```python
from build123d import *

# Parameters (mm, degrees)
CUT_EXTRUDE1_DEPTH = 3.5
CHAMFER1_SIZE      = 0.288675135
CHAMFER1_SIZE2     = 0.5


with BuildPart() as part:
    # Sketch1 → Revolve1 (revolve)
    with BuildSketch(Plane.XY, mode=Mode.PRIVATE) as revolve1_sk:
        Polygon((-20, 2), (-19, 3), (0, 3), (0, 0), (-20, 0), align=None)
    revolve(revolve1_sk.sketch.rotate(Axis((0, 0, 0), (-1, 0, 0)), 90), axis=Axis((0, 0, 0), (-1, 0, 0)))

    # Sketch2 → Cut-Extrude1 (cut)
    with BuildSketch(Plane(origin=(0, 0, 0), x_dir=(0, 0, -1), z_dir=(1, 0, 0))):
        Polygon((1.732050808, 0), (0.866025404, 1.5), (-0.866025404, 1.5), (-1.732050808, 0), (-0.866025404, -1.5), (0.866025404, -1.5), align=None)
    extrude(amount=-CUT_EXTRUDE1_DEPTH, mode=Mode.SUBTRACT)

    # Chamfer1
    chamfer1_edges = [part.edges().sort_by_distance(p)[0] for p in [
        (0, 0, 3),
    ]]
    chamfer1_side = [part.faces().sort_by_distance(p)[0] for p in [
        (-9.5, 0, 3),
    ]]
    chamfer(chamfer1_edges, length=CHAMFER1_SIZE, length2=CHAMFER1_SIZE2, reference=chamfer1_side[0])


solid = part.part
```
Could you check a few things on this model? Use its own coordinates, in mm. A direction names the side the tool comes from. Coordinates: 2 decimals unless noted, no trailing zeros. Write each loop counter-clockwise with the first axis right and the second up, starting at its lowest first coordinate (ties: lowest second). Pieces come first, ordered by that corner, then holes. Notation, with made-up numbers: (11.25, -6) -> (22.25, -6) arc R16 ccw to (22.25, 24) -> close; hole circle Ø1 at (71, 49.5). An arc over 180 degrees is marked (long way). Write item = value, one per line. Start each with the question number.
(1) We'd pull the mould along Z, two halves only. Please class faces 1 (the face through (0, 2, 0)), 2 (the face through (-9.51, -0.9, -2.86)), 3 (the face through (-1.726, 0.76, 1.293)): released by +Z, released by -Z, zero draft, split by the parting line, or undercut.
(2) Which directions (+Z, -Z, +X, -X, +Y, -Y) give clear straight access to the entire face, cutting with the end or side of a thin tool? Please do faces 4 (the face through (-20, 0, 0)), 5 (the face through (-2, -1.5, 0)).
(3) I want a section at C-C (x = -8.75). Please give me the cut outline in (y, z).
(4) I want a section at B-B (z = 0). Please give me the cut outline in (x, y), plus the area to 3 significant figures.
(5) I need wall thicknesses on line 1 (X direction, y = 0.25, z = -1.35); line 2 (Z direction, x = -2.25, y = -1.2); line 3 (Y direction, x = -3, z = -2.6). Which ranges of each line are inside material? Lowest first, please. Write a range as [from, to].
(6) I want a section at A-A (x = -2.25). Please give me the cut outline in (y, z).
(7) Will these pins go through, and if not, where does the flat tip stop? pin 1 (2 mm diameter, centred on x = -14, y = -1, fed in from +Z); pin 2 (0.9 mm diameter, centred on y = 0, z = -0.5, fed in from +X); pin 3 (0.5 mm diameter, centred on x = -2.5, z = 0.5, fed in from +Y); pin 4 (1.5 mm diameter, centred on x = -11.5, y = 1, fed in from -Z).
Result set:
q1.face_1 = zero draft
q1.face_2 = split by the parting line
q1.face_3 = undercut
q2.face_4 = +Z, -Z, -X, +Y, -Y
q2.face_5 = +X
q3.outline = circle Ø6 at (0, 0)
q4.outline = (-20, -2) -> (-19, -3) -> (-0.29, -3) -> (0, -2.5) -> (0, -1.5) -> (-3.5, -1.5) -> (-3.5, 1.5) -> (0, 1.5) -> (0, 2.5) -> (-0.29, 3) -> (-19, 3) -> (-20, 2) -> close
q4.area = 108 mm2
q5.line_1 = [-20, -3.5]
q5.line_2 = [-2.75, -1.04], [1.04, 2.75]
q5.line_3 = [-1.5, 1.5]
q6.outline = circle Ø6 at (0, 0); hole (-1.5, -0.87) -> (0, -1.73) -> (1.5, -0.87) -> (1.5, 0.87) -> (0, 1.73) -> (-1.5, 0.87) -> close
q7.pin_1 = 3
q7.pin_2 = -3.5
q7.pin_3 = 2.99
q7.pin_4 = -2.99
